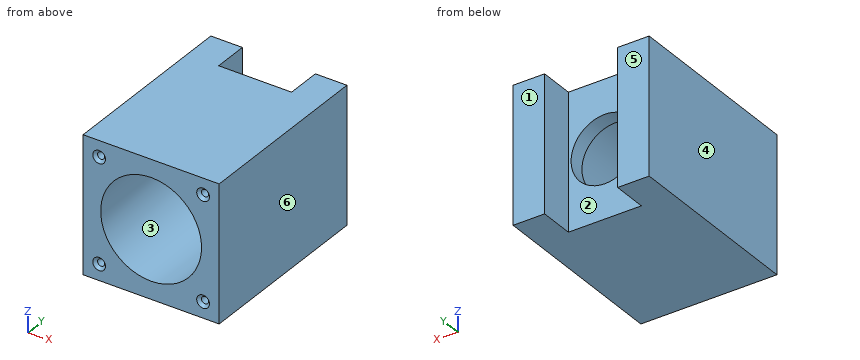
from build123d import *

# Parameters (mm, degrees)
SKETCH1_W                                = 30.43428
SKETCH1_H                                = 30.44952
BOSS_EXTRUDE1_DEPTH                      = 41.74236
SKETCH4_R                                = 7.5565
CUT_EXTRUDE3_DEPTH                       = 36.539424
SKETCH6_W                                = 16.31188
SKETCH6_H                                = 30.44952
CUT_EXTRUDE5_DEPTH                       = 7.75716
SKETCH8_R                                = 11.2776
CUT_EXTRUDE6_DEPTH                       = 30.44952
F_1_16_0_0625_DIAMETER_HOLE1_D           = 1.5875
F_1_16_0_0625_DIAMETER_HOLE1_DEPTH       = 12.7
F_1_16_0_0625_DIAMETER_HOLE1_CSINK_D     = 2.8575
F_1_16_0_0625_DIAMETER_HOLE1_CSINK_ANGLE = 90
F_1_16_0_0625_DIAMETER_HOLE1_TIP         = 0.476933116


with BuildPart() as part:
    # Sketch1 → Boss-Extrude1 (new body)
    with BuildSketch(Plane(origin=(0, 0, 0), x_dir=(1, 0, 0), z_dir=(0, 1, 0))):
        Rectangle(SKETCH1_W, SKETCH1_H)
    extrude(amount=BOSS_EXTRUDE1_DEPTH)

    # Sketch4 → Cut-Extrude3 (cut)
    with BuildSketch(Plane.XZ):
        with Locations(Location((0, 0, 0), (0, 0, 270))):
            Circle(SKETCH4_R)
    extrude(amount=-CUT_EXTRUDE3_DEPTH, mode=Mode.SUBTRACT)

    # Sketch6 → Cut-Extrude5 (cut)
    with BuildSketch(Plane(origin=(0, 41.74236, 0), x_dir=(1, 0, 0), z_dir=(0, 1, 0))):
        Rectangle(SKETCH6_W, SKETCH6_H)
    extrude(amount=-CUT_EXTRUDE5_DEPTH, mode=Mode.SUBTRACT)

    # Sketch8 → Cut-Extrude6 (cut)
    with BuildSketch(Plane.XZ):
        with Locations(Location((0, 0, 0), (0, 0, 270))):
            Circle(SKETCH8_R)
    extrude(amount=-CUT_EXTRUDE6_DEPTH, mode=Mode.SUBTRACT)

    # 1/16 (0.0625) Diameter Hole1
    with Locations(Plane(origin=(0, 0, 0), x_dir=(-1, 0, 0), z_dir=(0, -1, 0))):
        with Locations((-11.6205, 11.62812), (11.6205, 11.62812), (11.6205, -11.62812), (-11.6205, -11.62812)):
            CounterSinkHole(F_1_16_0_0625_DIAMETER_HOLE1_D / 2, F_1_16_0_0625_DIAMETER_HOLE1_CSINK_D / 2, depth=F_1_16_0_0625_DIAMETER_HOLE1_DEPTH, counter_sink_angle=F_1_16_0_0625_DIAMETER_HOLE1_CSINK_ANGLE)
            with Locations((0, 0, -(F_1_16_0_0625_DIAMETER_HOLE1_DEPTH + F_1_16_0_0625_DIAMETER_HOLE1_TIP / 2))):  # 118° drill point
                Cone(0, F_1_16_0_0625_DIAMETER_HOLE1_D / 2, F_1_16_0_0625_DIAMETER_HOLE1_TIP, mode=Mode.SUBTRACT)


solid = part.part
Geometry check sheet. Reference: the model listing, model coordinates, mm. Face numbers are marked on the shaded views. A direction names the side the tool comes from. Coordinates: 2 decimals unless noted, no trailing zeros. Order: outer loops, then holes, each group sorted by start corner. A loop starts at its lowest first (then second) coordinate and runs counter-clockwise, first axis right, second up. Notation, with made-up numbers: (34, -10.75) - (83, -10.75) arc R21 ccw to (83, 26.25) - close; hole circle Ø10 at (1.5, 19). An arc over 180 degrees is marked (long way). Answer in a Markdown table with one row per item. Add a question column.
1) Material ranges on line 1 along X through (y, z) = (18, 0); line 2 along X through (y, z) = (39, -11); line 3 along Y through (x, z) = (2, -9), recorded low to high. Write a range as [from, to].
2) Cross-section at A-A, the plane z = 0. Record the cut outline in (x, y).
3) Cross-section at C-C, the plane x = 0. Record the cut outline in (y, z).
4) Set-up check for the marked faces 1 and 2: record each of +Z, -Z, +X, -X, +Y, -Y from which the full face is reachable in a straight line by a thin tool's end or side.
5) Cross-section at D-D, the plane y = 17.5. Record the cut outline in (x, z).
6) Gauge pin test, flat end, axial feed: P1, Ø2.5, axis at x = -11.62, z = -11.63, coming from the -Y side. Record the tip position at first contact, or that the pin passes through.
7) Release check for a two-part mould opening along X. For the marked faces 3, 4, 5 and 6 record: +X half, -X half, draft (parallel to the pull), parting line (faces both ways), or undercut.
8) Cross-section at B-B, the plane y = 36. Record the cut outline in (x, z), then the cut area to 3 significant figures.
Check result:
| question | item | result |
|---|---|---|
| 1 | line 1 | x = [-15.22, -11.28], [11.28, 15.22] |
| 1 | line 2 | x = [-15.22, -8.16], [8.16, 15.22] |
| 1 | line 3 | y = [30.45, 33.99] |
| 2 | outline | (-15.22, 0) - (-11.28, 0) - (-11.28, 30.45) - (-7.56, 30.45) - (-7.56, 33.99) - (-8.16, 33.99) - (-8.16, 41.74) - (-15.22, 41.74) - close; (7.56, 30.45) - (11.28, 30.45) - (11.28, 0) - (15.22, 0) - (15.22, 41.74) - (8.16, 41.74) - (8.16, 33.99) - (7.56, 33.99) - close |
| 3 | outline | (0, -15.22) - (33.99, -15.22) - (33.99, -7.56) - (30.45, -7.56) - (30.45, -11.28) - (0, -11.28) - close; (0, 11.28) - (30.45, 11.28) - (30.45, 7.56) - (33.99, 7.56) - (33.99, 15.22) - (0, 15.22) - close |
| 4 | face 1 | +Z, -Z, +X, -X, +Y |
| 4 | face 2 | +Z, -Z, +Y |
| 5 | outline | (-15.22, -15.22) - (15.22, -15.22) - (15.22, 15.22) - (-15.22, 15.22) - close; hole circle Ø22.56 at (0, 0) |
| 6 | P1 | stops at y = 0.18 |
| 7 | face 3 | undercut |
| 7 | face 4 | -X half |
| 7 | face 5 | draft |
| 7 | face 6 | +X half |
| 8 | outline | (-15.22, -15.22) - (-8.16, -15.22) - (-8.16, 15.22) - (-15.22, 15.22) - close; (8.16, -15.22) - (15.22, -15.22) - (15.22, 15.22) - (8.16, 15.22) - close |
| 8 | area | 430 mm² |
